For this review, take the finished solid that the model builds, in its own axes (mm). A direction names the side the tool comes from. Give positions to 0.01 mm unless a question says otherwise; leave off trailing zeros. Write each loop counter-clockwise with the first axis right and the second up, starting at its lowest first coordinate (ties: lowest second). Pieces come first, ordered by that corner, then holes. Notation, with made-up numbers: (40.5, -38.5) -> (52.5, -38.5) arc R24 ccw to (52.5, -17.5) -> close; hole circle Ø2 at (30.25, 14). An arc over 180 degrees is marked (long way). Answer as CSV lines item,"result".
Autodesk Inventor part; units mm, degrees
ref_plane "YZ Plane" through (0, 0, 0) normal (1, 0, 0) x (0, 1, 0)
ref_plane "XZ Plane" through (0, 0, 0) normal (0, 1, 0) x (-1, 0, 0)
ref_plane "XY Plane" through (0, 0, 0) normal (0, 0, 1) x (1, 0, 0)
sketch "Sketch1" plane through (0, 0, 0) normal (0, 1, 0) x (-1, 0, 0)
  line L0 (-1.59, 12.5) -> (1.59, 12.5)
  line L1 (1.59, 12.5) -> (1.59, -12.5)
  line L2 (1.59, -12.5) -> (-1.59, -12.5)
  line L3 (-1.59, -12.5) -> (-1.59, 12.5)
  line L4 (-1.59, 12.5) -> (1.59, -12.5) construction
  line L5 (1.59, 12.5) -> (-1.59, -12.5) construction
  line L6 (12.5, 20) -> (-12.5, 20)
  line L7 (-12.5, 20) -> (-12.5, -20)
  line L8 (-12.5, -20) -> (12.5, -20)
  line L9 (12.5, -20) -> (12.5, 20)
  line L10 (12.5, 20) -> (107.5, 20)
  line L11 (107.5, 20) -> (107.5, -5)
  line L12 (107.5, -5) -> (12.5, -5)
  line L13 (12.5, -5) -> (12.5, 20)
  line L14 (107.5, 20) -> (82.5, 20)
  line L15 (88.91, 20) -> (92.09, 20)
  line L16 (102.5, 9.09) -> (87.5, 9.09)
  line L17 (87.5, 9.09) -> (87.5, 5.91)
  line L18 (87.5, 5.91) -> (102.5, 5.91)
  line L19 (102.5, 5.91) -> (102.5, 9.09)
  line L20 (96.59, 15) -> (93.41, 15)
  line L21 (93.41, 15) -> (93.41, 0)
  line L22 (93.41, 0) -> (96.59, 0)
  line L23 (96.59, 0) -> (96.59, 15)
  line L24 (96.59, 15) -> (93.41, 0) construction
  line L25 (93.41, 15) -> (96.59, 0) construction
  line L26 (50, 9.09) -> (35, 9.09)
  line L27 (35, 9.09) -> (35, 5.91)
  line L28 (35, 5.91) -> (50, 5.91)
  line L29 (50, 5.91) -> (50, 9.09)
  line L30 (44.09, 15) -> (40.91, 15)
  line L31 (40.91, 15) -> (40.91, 0)
  line L32 (40.91, 0) -> (44.09, 0)
  line L33 (44.09, 0) -> (44.09, 15)
  line L34 (44.09, 15) -> (40.91, 0) construction
  line L35 (40.91, 15) -> (44.09, 0) construction
  point P0 (0, 0)
  point P1 (95, 7.5)
  point P2 (42.5, 7.5)
  dimension "d0" = 3.18
  dimension "d1" = 25
  dimension "d2" = 25
  dimension "d3" = 12.5
  dimension "d4" = 20
  dimension "d5" = 20
  dimension "d6" = 95
  dimension "d7" = 25
  dimension "d35" = 15
  dimension "d36" = 3.18
  dimension "d38" = 3.18
  dimension "d39" = 15
  dimension "d40" = 7.5
  dimension "d41" = 1.59
  dimension "d42" = 12.5
  dimension "d43" = 12.5
  dimension "d44" = 15
  dimension "d45" = 3.18
  dimension "d46" = 3.18
  dimension "d47" = 15
  dimension "d48" = 7.5
  dimension "d49" = 1.59
  dimension "d50" = 30
  dimension "d51" = 12.5
extrude "Extrusion2" add sketch "Sketch1" along normal blind 3.18
properties part number "Brazo_Inferior"
Q1. Draft analysis for pull direction X (two halves, no side actions). For faces 1 (the flat face through (-47, 2, 9.09)), 2 (the flat face through (-107.5, 2, 8)), 3 (the flat face through (-61, 2, -5)), 4 (the flat face through (12.5, 2, 0)), state which applies: released by +X, released by -X, zero draft, split by the parting line, or undercut.
Answer block:
face 1,"undercut"
face 2,"released by -X"
face 3,"zero draft"
face 4,"released by +X"
Q2. Add section B-B (y = 1.8). State how many separate pieces and enclosed holes the cut face has, plus the area to 3 significant figures.
Answer block:
separate pieces,"1"
enclosed holes,"3"
area,"3,120 mm2"
Q3. Add section C-C (z = -10). Write out the cut boundary in (x, y).
Answer block:
outline,"(-12.5, 0) -> (-1.59, 0) -> (-1.59, 3.18) -> (-12.5, 3.18) -> close; (1.59, 0) -> (12.5, 0) -> (12.5, 3.18) -> (1.59, 3.18) -> close"
Q4. To check wall thickness, follow probe 1 along X at (y, z) = (0.5, 2); probe 2 along X at (y, z) = (2, 14.5); probe 3 along X at (y, z) = (2, 8.5). State the ranges of each line that lie inside material, in increasing order. Write a range as [from, to].
Answer block:
probe 1,"x = [-107.5, -96.59], [-93.41, -44.09], [-40.91, -1.59], [1.59, 12.5]"
probe 2,"x = [-107.5, -96.59], [-93.41, -44.09], [-40.91, 12.5]"
probe 3,"x = [-107.5, -102.5], [-87.5, -50], [-35, -1.59], [1.59, 12.5]"
Q5. Clearance check with a flat-ended pin moving along its axis: pin 1 (1 mm diameter, centred on x = -38, y = 1, fed in from -Z). State where the tip first meets the part, or that it passes through.
Answer block:
pin 1,"stops at z = -5"
Q6. Add section D-D (x = -74). Write out the cut boundary in (y, z).
Answer block:
outline,"(0, -5) -> (3.18, -5) -> (3.18, 20) -> (0, 20) -> close"
Q7. For faces 5 (the flat face through (0, 2, -20)), 6 (the flat face through (-90, 2, 5.91)), list the 3-axis set-ups (+Z, -Z, +X, -X, +Y, -Y) from which the entire face can be reached by the end or side of a thin tool; tool diameter is ignored.
Answer block:
face 5,"-Z, +X, -X, +Y, -Y"
face 6,"+Y, -Y"
Q8. Add section A-A (z = -1.5). Write out the cut boundary in (x, y).
Answer block:
outline,"(-107.5, 0) -> (-1.59, 0) -> (-1.59, 3.18) -> (-107.5, 3.18) -> close; (1.59, 0) -> (12.5, 0) -> (12.5, 3.18) -> (1.59, 3.18) -> close"
